```python
from build123d import *

# Parameters (mm, degrees)
F1_DEPTH = 9


with BuildPart() as f1:
    # F0 (on Top) → F1 (new body)
    with BuildSketch(Plane.XY):
        with BuildLine():
            Line((-45, 0), (0, 0))
            Line((0, 0), (0, 2))
            Line((0, 2), (3, 2))
            Line((3, 2), (3, 0))
            Line((3, 0), (28, 0))
            Line((28, 0), (28, 2))
            Line((28, 2), (23.403733, 5.856726))
            Line((23.403733, 5.856726), (16.403733, 5.856726))
            ThreePointArc((16.403733, 5.856726), (11.903733, 3), (7.403733, 5.856726))
            Line((7.403733, 5.856726), (-4.596267, 5.856726))
            ThreePointArc((-4.596267, 5.856726), (-6.096267, 5), (-7.596267, 5.856726))
            Line((-7.596267, 5.856726), (-12.596267, 5.856726))
            ThreePointArc((-12.596267, 5.856726), (-15.596267, 4), (-18.596267, 5.856726))
            Line((-18.596267, 5.856726), (-45, 0))
        make_face()
    extrude(amount=F1_DEPTH)


solid = f1.part
```
Work out the finished part from the listing and answer in its coordinate system (mm). A direction names the side the tool comes from. Give positions to 0.01 mm unless a question says otherwise; leave off trailing zeros. Loops run counter-clockwise (first coordinate to the right, second up) from the corner with the lowest first, then second, coordinate; pieces in that order, holes last. Notation, with made-up numbers: (20, 44) -> (73, 44) arc R31 ccw to (73, 76) -> close; hole circle Ø7 at (81.5, 29.25). An arc over 180 degrees is marked (long way). One line per question, with ' | ' between items. Start each with the question number.
1) Section D-D, the plane x = 14 is taken. Determine the outline of the cut face in (y, z).
2) Section B-B, the plane y = 0.6 is taken. Determine the outline of the cut face in (x, z).
3) For faces 1 (the face through (1, 5.857, 4)), 2 (the face through (1, 2, 4)), determine the directions among +Z, -Z, +X, -X, +Y, -Y from which every point of the face is accessible in a straight line to the end or side of a thin tool.
4) Straight lines are drawn through the part: L1, parallel to Y at x = -22.5, z = 3.25; L2, parallel to Y at x = -27, z = 4.25. For each, find the intervals that lie inside material, in ascending order.
5) Each of these flat-tipped pins is pushed along its axis until it touches: pin 1 (2 mm diameter, centred on x = -23, z = 5.5, fed in from -Y); pin 2 (0.9 mm diameter, centred on x = 2, z = 6.5, fed in from -Y); pin 3 (3 mm diameter, centred on x = -32, z = 7.5, fed in from +Y). Where does it stop, or does it pass through?
6) Determine the mould class of faces 3 (the face through (25.734, 3.901, 4.437)), 4 (the face through (12, 3, 4)), 5 (the face through (-23, 0, 4)), 6 (the face through (-15.5, 4, 4.4)) for opening direction X: +X half, -X half, draft (parallel to the pull), parting line (faces both ways), or undercut.
7) Section C-C, the plane x = 1.5 is taken. Determine the outline of the cut face in (y, z).
8) Section A-A, the plane z = 6.75 is taken. Determine the outline of the cut face in (x, y), then the cut area to 3 significant figures.
Resolved:
1) outline: (0, 0) -> (3.46, 0) -> (3.46, 9) -> (0, 9) -> close
2) outline: (-42.3, 0) -> (0, 0) -> (0, 9) -> (-42.3, 9) -> close; (3, 0) -> (28, 0) -> (28, 9) -> (3, 9) -> close
3) face 1: +Z, -Z, +X, -X, +Y | face 2: +Z, -Z, -Y
4) L1: 0 to 4.99 | L2: 0 to 3.99
5) pin 1: y = 0 | pin 2: y = 2 | pin 3: y = 3.22
6) face 3: +X half | face 4: undercut | face 5: draft | face 6: undercut
7) outline: (2, 0) -> (5.86, 0) -> (5.86, 9) -> (2, 9) -> close
8) outline: (-45, 0) -> (0, 0) -> (0, 2) -> (3, 2) -> (3, 0) -> (28, 0) -> (28, 2) -> (23.4, 5.86) -> (16.4, 5.86) arc R4.97 cw to (7.4, 5.86) -> (-4.6, 5.86) arc R1.74 cw to (-7.6, 5.86) -> (-12.6, 5.86) arc R3.35 cw to (-18.6, 5.86) -> close | area: 307 mm2
